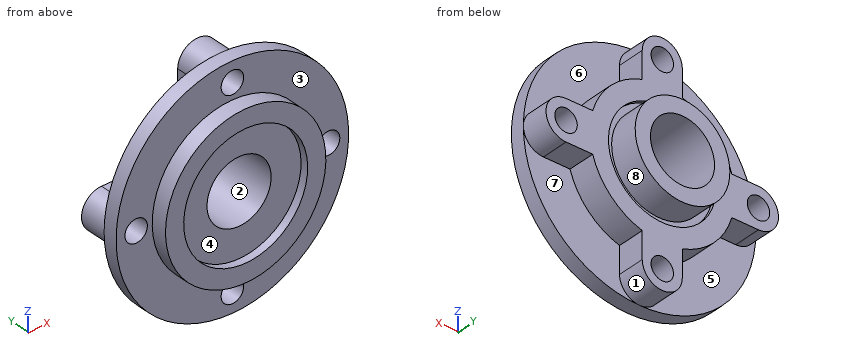
Solid Edge part; units mm, degrees
sketch "Sketch1" plane through (0, 0, 0) normal (1, 0, 0) x (0, 1, 0)
  line L0 (-16.4856, 20) -> (29.747, 20)
  line L1 (29.747, 20) -> (29.747, 29.5367)
  line L2 (29.747, 29.5367) -> (12.0813, 29.5367)
  line L3 (12.0813, 33.5455) -> (12.0813, 29.5367)
  line L4 (14.547, 33.5455) -> (12.0813, 33.5455)
  line L5 (14.547, 33.5455) -> (14.547, 45.137)
  line L6 (14.547, 45.137) -> (-2.453, 45.137)
  line L7 (-2.453, 45.137) -> (-2.453, 72.5)
  line L8 (-2.453, 72.5) -> (-11.453, 72.5)
  line L9 (-11.453, 72.5) -> (-11.453, 50)
  line L10 (-11.453, 50) -> (-21.453, 50)
  line L11 (-21.453, 50) -> (-21.453, 38.6647)
  line L12 (-21.453, 38.6647) -> (-16.4856, 38.6647)
  line L13 (-16.4856, 38.6647) -> (-16.4856, 20)
revolve "RevolvedProtrusion1" add sketch "Sketch1" angle 360 about axis through (0, -60, 0) along (0, 1, 0)
sketch "Sketch2" plane through (0, 14.547, 0) normal (0, 1, 0) x (-1, 0, 0)
  line L0 (-12.5, 43.3717) -> (-12.5, 60)
  arc A0 (-12.5, 60) -> (12.5, 60) centre (0, 60) cw
  line L1 (12.5, 60) -> (12.5, 43.3717)
  arc A1 (-12.5, 43.3717) -> (12.5, 43.3717) centre (0, 0) cw
extrude "Protrusion1" add sketch "Sketch2" against normal up to next
hole "Hole1" at (0, 14.547, 60) direction (0, -1, 0) diameter 14 end up to next
pattern_circular "Pattern1" count 4 over 360 about axis through (0, 0, 0) along (0, 1, 0) of "Protrusion1"
pattern_circular "Pattern2" count 4 over 360 about axis through (0, 14.547, 0) along (0, -1, 0) of "Hole1"
Read the model definition and answer for the solid it produces. Units are mm, in the model's axes. Face numbers are marked on the shaded views. A direction names the side the tool comes from. Round coordinates to 2 decimals unless told otherwise and drop trailing zeros. Write each loop counter-clockwise with the first axis right and the second up, starting at its lowest first coordinate (ties: lowest second). Pieces come first, ordered by that corner, then holes.
Q1. Straight lines are drawn through the part: line 1 (X direction, y = 3.75, z = 0); line 2 (X direction, y = -13.5, z = -0.5); line 3 (Z direction, x = -60, y = 0). For each, find the intervals that lie inside material, in ascending order.
Values:
line 1: x = -72.5 to -67, -53 to -20, 20 to 53, 67 to 72.5
line 2: x = -50 to -19.99, 19.99 to 50
line 3: z = -12.5 to -7, 7 to 12.5
Q2. A tool of negligible diameter and unlimited length cuts with its end or side. For the marked faces 4, 5, 6, 7 and 8, from which of +Z, -Z, +X, -X, +Y, -Y can it reach the whole face along a straight path? Write none if from no direction.
Values:
face 4: -Y
face 5: -Z, -X, +Y
face 6: +Z, +X, +Y
face 7: -Z, +X, +Y
face 8: +Y
Q3. The mould has two halves that part along X. Classify the marked faces 1, 2 and 3: released by +X, released by -X, zero draft, split by the parting line, or undercut.
Values:
face 1: split by the parting line
face 2: undercut
face 3: zero draft
Q4. Find section D-D on x = 27. Determine the outline of the cut face in (y, z).
Values:
outline: (-21.45, -42.08) - (-11.45, -42.08) - (-11.45, -67.28) - (-2.45, -67.28) - (-2.45, -36.17) - (14.55, -36.17) - (14.55, -19.91) - (12.08, -19.91) - (12.08, -11.98) - (29.75, -11.98) - (29.75, 11.98) - (12.08, 11.98) - (12.08, 19.91) - (14.55, 19.91) - (14.55, 36.17) - (-2.45, 36.17) - (-2.45, 67.28) - (-11.45, 67.28) - (-11.45, 42.08) - (-21.45, 42.08) - (-21.45, 27.68) - (-16.49, 27.68) - (-16.49, -27.68) - (-21.45, -27.68) - close
Q5. Find section A-A on y = 6.5. Determine the outline of the cut face in (x, z).
Values:
outline: (-60, -12.5) - (-43.37, -12.5) arc R45.14 ccw to (-12.5, -43.37) - (-12.5, -60) arc R12.5 ccw to (12.5, -60) - (12.5, -43.37) arc R45.14 ccw to (43.37, -12.5) - (60, -12.5) arc R12.5 ccw to (60, 12.5) - (43.37, 12.5) arc R45.14 ccw to (12.5, 43.37) - (12.5, 60) arc R12.5 ccw to (-12.5, 60) - (-12.5, 43.37) arc R45.14 ccw to (-43.37, 12.5) - (-60, 12.5) arc R12.5 ccw to start; hole circle Ø14 at (-60, 0); hole circle Ø40 at (0, 0); hole circle Ø14 at (0, -60); hole circle Ø14 at (0, 60); hole circle Ø14 at (60, 0)
Q6. Find section B-B on x = -58. Determine the outline of the cut face in (y, z), and give its area (3 significant figures).
Values:
outline: (-11.45, -43.5) - (-2.45, -43.5) - (-2.45, -12.5) - (14.55, -12.5) - (14.55, -6.71) - (-11.45, -6.71) - close; (-11.45, 6.71) - (14.55, 6.71) - (14.55, 12.5) - (-2.45, 12.5) - (-2.45, 43.5) - (-11.45, 43.5) - close
area: 859 mm2
Q7. Flat-ended cylindrical pins translate along their axes: P1, Ø10, axis at x = -56, z = -16, coming from the -Y side; P2, Ø8, axis at y = 0, z = 0.5, coming from the -X side; P3, Ø5, axis at y = 7, z = 48, coming from the -X side; P4, Ø8.5, axis at x = -54, y = 6, coming from the -Z side. Find the tip coordinate at first contact, or state that the pin passes through.
Values:
P1: stops at y = -11.45
P2: stops at x = -72.5
P3: stops at x = -12.5
P4: stops at z = -12.5
Q8. Find section C-C on z = -48. Determine the outline of the cut face in (x, y), and give its area (3 significant figures).
Values:
outline: (-54.33, -11.45) - (-14, -11.45) - (-14, -21.45) - (14, -21.45) - (14, -11.45) - (54.33, -11.45) - (54.33, -2.45) - (12.5, -2.45) - (12.5, 14.55) - (-12.5, 14.55) - (-12.5, -2.45) - (-54.33, -2.45) - close
area: 1,680 mm2
